Study the drawing (mm; zero at the part's minimum x, y, z) and answer. Give positions to 0.01 mm unless a question says otherwise; leave off trailing zeros. Write each loop counter-clockwise with the first axis right and the second up, starting at its lowest first coordinate (ties: lowest second). Pieces come first, ordered by that corner, then holes. Notation, with made-up numbers: (64, 21.5) - (111, 21.5) arc R15 cw to (111, 40.5) - close; hole circle Ø11 at (82, 56.25). An arc over 180 degrees is marked (long way). Write each question's results on one line, items separated by ' | '. Start each with the question number.
Q1. Section A-A (x = 26) is taken. Determine the outline of the cut face in (y, z) (1 decimal).
Q2. A flat-ended cylindrical pin translates along its axis: pin 1 Ø1.8 at (x, y) = (43.58, 31.91) entering from +Z. Find the tip coordinate at first contact, or state that the pin passes through.
Q3. Section C-C (x = 13.5) is taken. Determine the outline of the cut face in (y, z).
Q4. Section B-B (y = 18.5) is taken. Determine the outline of the cut face in (x, z), plus the area to 3 significant figures.
Q5. Section D-D (z = 2.45) is taken. Determine the outline of the cut face in (x, y) (1 decimal), plus the area to 3 significant figures.
Q6. Find the intervals of material crossed by probe 1 along Y at (x, z) = (27.5, 0.6) (1 decimal); probe 2 along Y at (x, z) = (21.5, 1.55); probe 3 along X at (y, z) = (10, 0.45) (1 decimal), in increasing order.
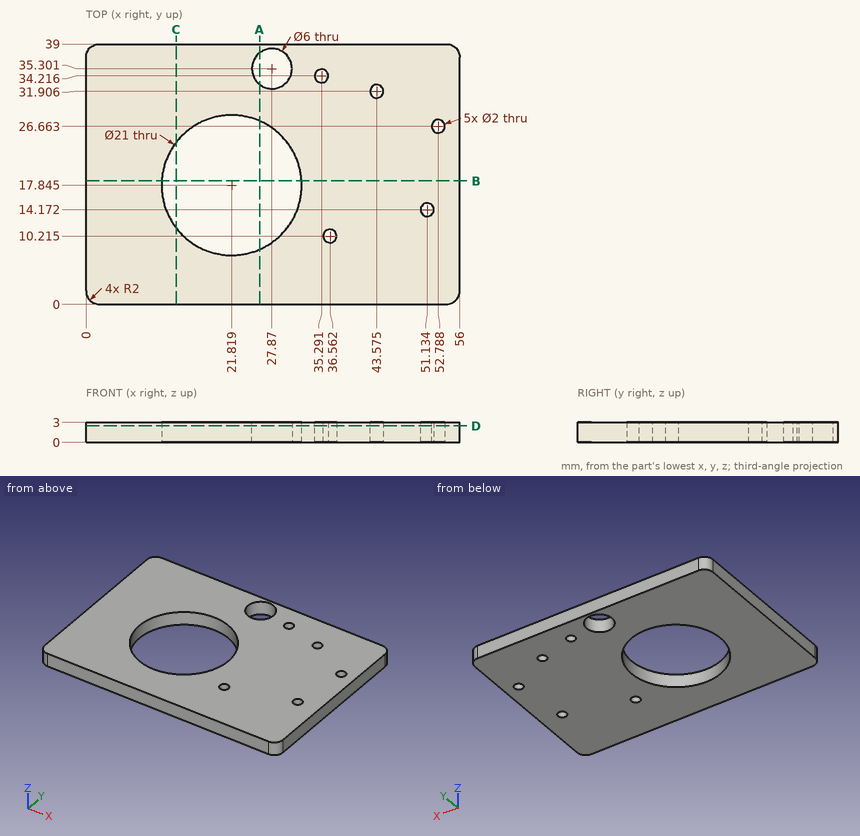
Answers below:
1) outline: (0, 0) - (8.2, 0) - (8.2, 3) - (0, 3) - close; (27.5, 0) - (33, 0) - (33, 3) - (27.5, 3) - close; (37.6, 0) - (39, 0) - (39, 3) - (37.6, 3) - close
2) pin 1: passes through
3) outline: (0, 0) - (11.44, 0) - (11.44, 3) - (0, 3) - close; (24.25, 0) - (39, 0) - (39, 3) - (24.25, 3) - close
4) outline: (0, 0) - (11.34, 0) - (11.34, 3) - (0, 3) - close; (32.3, 0) - (56, 0) - (56, 3) - (32.3, 3) - close | area: 105 mm2
5) outline: (0, 2) arc R2 ccw to (2, 0) - (54, 0) arc R2 ccw to (56, 2) - (56, 37) arc R2 ccw to (54, 39) - (2, 39) arc R2 ccw to (0, 37) - close; hole circle Ø21 at (21.8, 17.8); hole circle Ø6 at (27.9, 35.3); hole circle Ø2 at (35.3, 34.2); hole circle Ø2 at (36.6, 10.2); hole circle Ø2 at (43.6, 31.9); hole circle Ø2 at (51.1, 14.2); hole circle Ø2 at (52.8, 26.7) | area: 1,790 mm2
6) probe 1: y = 0 to 9, 26.7 to 32.3, 38.3 to 39 | probe 2: y = 0 to 7.35, 28.34 to 39 | probe 3: x = 0 to 14.8, 28.8 to 35.6, 37.5 to 56
